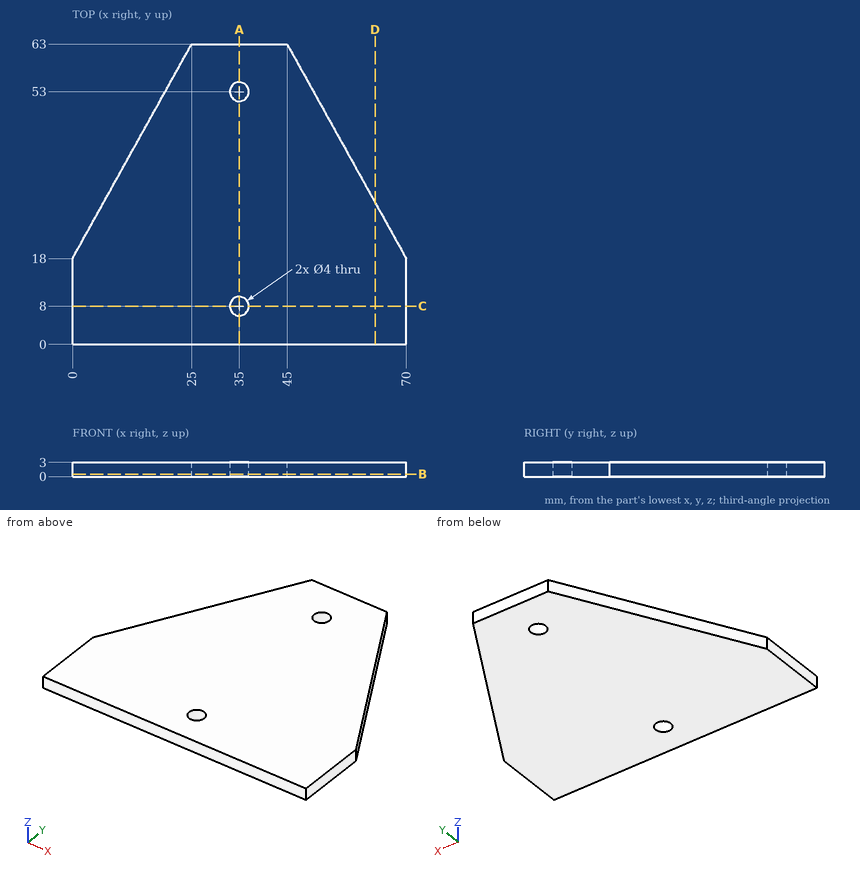
Design review of the part shown in the three views and the two pictorial views. Dimensions are in mm from the part's minimum x, y and z. Round coordinates to 2 decimals unless told otherwise and drop trailing zeros. Loops run counter-clockwise (first coordinate to the right, second up) from the corner with the lowest first, then second, coordinate; pieces in that order, holes last. Notation, with made-up numbers: M -11,78.25 L 42,78.25 A10 ccw 42,90.25 Z; hole C 4.5,17 d4. An arc over 180 degrees is marked long. Put each result on its own line as item: value.
Q1. To check wall thickness, follow L1, parallel to Y at x = 35, z = 1.7; L2, parallel to Y at x = 35.5, z = 1.95; L3, parallel to Y at x = 21.5, z = 1.75. State the ranges of each line that lie inside material, in increasing order.
Result set:
L1: y = 0 to 6, 10 to 51, 55 to 63
L2: y = 0 to 6.06, 9.94 to 51.06, 54.94 to 63
L3: y = 0 to 56.7
Q2. Consider section C-C, the plane y = 8. Give the boundary of the cut face in (x, z), then the cut area to 3 significant figures.
Result set:
outline: M 0,0 L 33,0 L 33,3 L 0,3 Z; M 37,0 L 70,0 L 70,3 L 37,3 Z
area: 198 mm²
Q3. For pin 1 (2.5 mm diameter, centred on x = 35, y = 8, fed in from +Z); pin 2 (10 mm diameter, centred on x = 28, y = 32.5, fed in from -Z), all flat-tipped, find the tip position at first contact; note any pin that passes through.
Result set:
pin 1: passes through
pin 2: stops at z = 0
Q4. Consider section A-A, the plane x = 35. Give the boundary of the cut face in (y, z), then the cut area to 3 significant figures.
Result set:
outline: M 0,0 L 6,0 L 6,3 L 0,3 Z; M 10,0 L 51,0 L 51,3 L 10,3 Z; M 55,0 L 63,0 L 63,3 L 55,3 Z
area: 165 mm²
Q5. Consider section D-D, the plane x = 63.5. Give the boundary of the cut face in (y, z), then the cut area to 3 significant figures.
Result set:
outline: M 0,0 L 29.7,0 L 29.7,3 L 0,3 Z
area: 89.1 mm²
Q6. Consider section B-B, the plane z = 0.5. Give the boundary of the cut face in (x, y), then the cut area to 3 significant figures.
Result set:
outline: M 0,0 L 70,0 L 70,18 L 45,63 L 25,63 L 0,18 Z; hole C 35,8 d4; hole C 35,53 d4
area: 3,260 mm²
